Solid Edge part; units mm, degrees
sketch "Sketch1" plane through (0, 0, 0) normal (0, -1, 0) x (1, 0, 0)
  line L0 (-47, -47) -> (47, -47)
  line L1 (47, -47) -> (47, 47)
  line L2 (47, 47) -> (-47, 47)
  line L3 (-47, 47) -> (-47, -47)
extrude "Protrusion1" add sketch "Sketch1" against normal blind 1.2
sketch "Sketch2" plane through (0, 1.2, 0) normal (0, 1, 0) x (0, 0, -1)
  line L0 (-31.0077, 45.5) -> (-31.0077, 33.4066)
  line L1 (-31.0077, 33.4066) -> (-46, 33.4066)
  line L2 (-46, 33.4066) -> (-46, -38.6606)
  line L3 (-46, -38.6606) -> (-35.6145, -38.6606)
  line L4 (-35.6145, -38.6606) -> (-35.6145, -45.5)
  line L5 (-35.6145, -45.5) -> (33.5653, -45.5)
  line L6 (33.5653, -45.5) -> (33.5653, -38.5694)
  line L7 (33.5653, -38.5694) -> (46, -38.5694)
  line L8 (46, -38.5694) -> (46, 34.0082)
  line L9 (46, 34.0082) -> (30.5923, 34.0082)
  line L10 (30.5923, 34.0082) -> (30.5923, 44.4526)
  line L11 (30.5923, 45.5) -> (30.5923, 44.4526)
  line L12 (-31.0077, 45.5) -> (30.5923, 45.5)
  dimension "D1" = 31.0077
  dimension "D2" = 46
  dimension "D3" = 35.6145
  dimension "D4" = 33.5653
  dimension "D5" = 46
extrude "Cutout1" cut sketch "Sketch2" along normal mid plane 166.709 flip side to cut
sketch "Sketch3" plane through (0, 0, 0) normal (0, -1, 0) x (0, 0, 1)
  circle A0 centre (28, 0) radius 1.25
extrude "ExtrudedCutout_4" cut sketch "Sketch3" along normal mid plane 57.9991
sketch "Sketch4" plane through (0, 0, 0) normal (0, -1, 0) x (0, 0, 1)
  circle A0 centre (-28, 0) radius 1.25
extrude "ExtrudedCutout_5" cut sketch "Sketch4" along normal mid plane 49.1039
properties material "Epoxy, cast rigid"
CAD build for the part. Positions are in the model's coordinates, mm. Round coordinates to 2 decimals unless told otherwise and drop trailing zeros. Write each loop counter-clockwise with the first axis right and the second up, starting at its lowest first coordinate (ties: lowest second). Pieces come first, ordered by that corner, then holes. Notation, with made-up numbers: (38, 48.25) -> (73, 48.25) arc R35 cw to (73, 81.25) -> close; hole circle Ø5 at (84, 60.25). An arc over 180 degrees is marked (long way). Answer in a Markdown table with one row per item. Add a question column.
Item 1: Mould opens along X. For faces 1 (the face through (1, 1.2, 1)), 2 (the face through (0.479, 0.592, 29.155)) say: pulls with the +X half, pulls with the -X half, needs draft (parallel to the pull), parting line crosses it, or undercut.
Item 2: Saw through at D-D, the plane x = -36. Write the cut outline in (y, z).
Item 3: Saw through at A-A, the plane z = 28. Write the cut outline in (x, y), then the cut area to 3 significant figures.
Item 4: Drop a flat-ended pin along its axis: pin 1 Ø0.6 at (y, z) = (0.5, 38.5) entering from -X. Give the stop position or say it passes through.
Item 5: Saw through at B-B, the plane x = 0. Write the cut outline in (y, z), then the cut area to 3 significant figures.
Item 6: Saw through at C-C, the plane y = 1. Write the cut outline in (x, z), then the cut area to 3 significant figures.
Item 7: Drill centre lines: line 1 (Z direction, x = 0, y = 0.45); line 2 (X direction, y = 0.85, z = -28); line 3 (Z direction, x = 41, y = 0.2). Where is each one in solid material? Low to high. Write a range as from..to.
Findings below:
| question | item | result |
|---|---|---|
| 1 | face 1 | needs draft |
| 1 | face 2 | undercut |
| 2 | outline | (0, -30.59) -> (1.2, -30.59) -> (1.2, 31.01) -> (0, 31.01) -> close |
| 3 | outline | (-45.5, 0) -> (-1.25, 0) -> (-1.25, 1.2) -> (-45.5, 1.2) -> close; (1.25, 0) -> (45.5, 0) -> (45.5, 1.2) -> (1.25, 1.2) -> close |
| 3 | area | 106 mm^2 |
| 4 | pin 1 | stops at x = -33.41 |
| 5 | outline | (0, -46) -> (1.2, -46) -> (1.2, -29.25) -> (0, -29.25) -> close; (0, -26.75) -> (1.2, -26.75) -> (1.2, 26.75) -> (0, 26.75) -> close; (0, 29.25) -> (1.2, 29.25) -> (1.2, 46) -> (0, 46) -> close |
| 5 | area | 104 mm^2 |
| 6 | outline | (-45.5, -30.59) -> (-34.01, -30.59) -> (-34.01, -46) -> (38.57, -46) -> (38.57, -33.57) -> (45.5, -33.57) -> (45.5, 35.61) -> (38.66, 35.61) -> (38.66, 46) -> (-33.41, 46) -> (-33.41, 31.01) -> (-45.5, 31.01) -> close; hole circle Ø2.5 at (0, -28); hole circle Ø2.5 at (0, 28) |
| 6 | area | 7,850 mm^2 |
| 7 | line 1 | z = -46..-29.25, -26.75..26.75, 29.25..46 |
| 7 | line 2 | x = -45.5..-1.25, 1.25..45.5 |
| 7 | line 3 | z = -33.57..35.61 |
